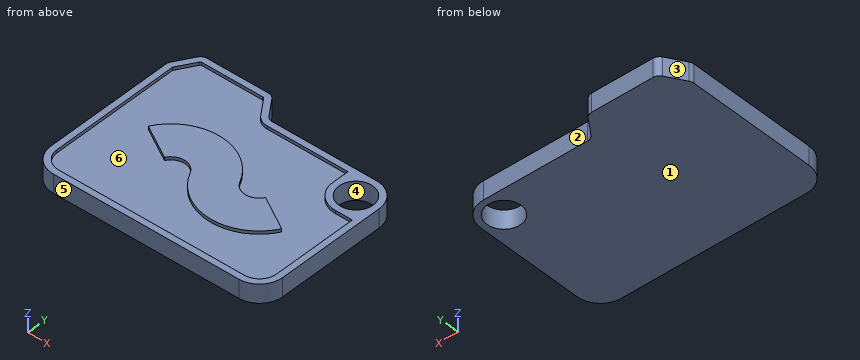
from build123d import *

# Parameters (mm, degrees)
F0_R     = 2.1999998258
F1_DEPTH = 2
F2_DEPTH = 0.4


# Not quite as in the source:
# - ends of sketch curves that miss each other by under 0.0002 mm in the source are joined


with BuildPart() as f1:
    # F0 (on Top) → F1 (new body)
    with BuildSketch(Plane.XY):
        with BuildLine():
            Line((12, 10), (-1.4882636307, 10))
            ThreePointArc((-1.4882636307, 10), (-1.9438159565, 10.1097909917), (-2.2993371991, 10.4150558431))
            Line((-2.2993371991, 10.4150558431), (-3.8642550313, 12.5849441569))
            ThreePointArc((-3.8642550313, 12.5849441569), (-4.2197762739, 12.8902090083), (-4.6753285997, 13))
            Line((-4.6753285997, 13), (-12.6032477109, 13))
            ThreePointArc((-12.6032477109, 13), (-13.0920798627, 12.8723778582), (-13.456140402, 12.5220862548))
            Line((-13.456140402, 12.5220862548), (-14.8528926911, 10.2403180459))
            ThreePointArc((-14.8528926911, 10.2403180459), (-14.9625208286, 9.989439561), (-15, 9.7182317911))
            Line((-15, 9.7182317911), (-15, -7))
            ThreePointArc((-15, -7), (-14.1213203436, -9.1213203436), (-12, -10))
            Line((-12, -10), (12, -10))
            ThreePointArc((12, -10), (14.1213203436, -9.1213203436), (15, -7))
            Line((15, -7), (15, 7))
            ThreePointArc((15, 7), (14.1213203436, 9.1213203436), (12, 10))
        make_face()
        with BuildLine():
            ThreePointArc((-14.1999998258, 9.7182317911), (-14.192503998, 9.7724732978), (-14.1705783896, 9.8226489511))
            Line((-14.1705783896, 9.8226489511), (-12.7738261005, 12.10441716))
            ThreePointArc((-12.7738261005, 12.10441716), (-12.7010140561, 12.1744754196), (-12.6032477109, 12.1999998258))
            Line((-12.6032477109, 12.1999998258), (-4.6753285997, 12.1999998258))
            ThreePointArc((-4.6753285997, 12.1999998258), (-4.5842182139, 12.1780416465), (-4.5131140273, 12.1169887295))
            Line((-4.5131140273, 12.1169887295), (-2.9481961951, 9.9471004156))
            ThreePointArc((-2.9481961951, 9.9471004156), (-2.3082578965, 9.3976236299), (-1.4882636307, 9.1999998258))
            Line((-1.4882636307, 9.1999998258), (9.0000001742, 9.1999998258))
            Line((9.0000001742, 9.1999998258), (9.0000001742, 7))
            ThreePointArc((9.0000001742, 7), (9.8786797797, 4.8786797797), (12, 4.0000001742))
            Line((12, 4.0000001742), (14.1999998258, 4))
            Line((14.1999998258, 4), (14.1999998258, -7))
            ThreePointArc((14.1999998258, -7), (13.5556347954, -8.5556347954), (12, -9.1999998258))
            Line((12, -9.1999998258), (-12, -9.1999998258))
            ThreePointArc((-12, -9.1999998258), (-13.5556347954, -8.5556347954), (-14.1999998258, -7))
            Line((-14.1999998258, -7), (-14.1999998258, 9.7182317911))
        make_face(mode=Mode.SUBTRACT)
        with Locations((12, 7)):
            Circle(F0_R, mode=Mode.SUBTRACT)
        with BuildLine():
            Line((-12.7738261005, 12.10441716), (-14.1705783896, 9.8226489511))
            ThreePointArc((-14.1705783896, 9.8226489511), (-14.192503998, 9.7724732978), (-14.1999998258, 9.7182317911))
            Line((-14.1999998258, 9.7182317911), (-14.1999998258, -7))
            ThreePointArc((-14.1999998258, -7), (-13.5556347954, -8.5556347954), (-12, -9.1999998258))
            Line((-12, -9.1999998258), (12, -9.1999998258))
            ThreePointArc((12, -9.1999998258), (13.5556347954, -8.5556347954), (14.1999998258, -7))
            Line((14.1999998258, -7), (14.1999998258, 4))
            Line((14.1999998258, 4), (12, 4))
            ThreePointArc((12, 4), (9.8786797797, 4.8786797797), (9.0000001742, 7))
            Line((9.0000001742, 7), (9.0000001742, 9.1999998258))
            Line((9.0000001742, 9.1999998258), (-1.4882636307, 9.1999998258))
            ThreePointArc((-1.4882636307, 9.1999998258), (-2.3082578965, 9.3976236299), (-2.9481961951, 9.9471004156))
            Line((-2.9481961951, 9.9471004156), (-4.5131140273, 12.1169887295))
            ThreePointArc((-4.5131140273, 12.1169887295), (-4.5842182139, 12.1780416465), (-4.6753285997, 12.1999998258))
            Line((-4.6753285997, 12.1999998258), (-12.6032477109, 12.1999998258))
            ThreePointArc((-12.6032477109, 12.1999998258), (-12.7010140561, 12.1744754196), (-12.7738261005, 12.10441716))
        make_face()
        with BuildLine():
            ThreePointArc((10, -1.5313274312), (3.7431454959, -4.9955321683), (-2.2491392669, -1.0915001412))
            ThreePointArc((-2.2491392669, -1.0915001412), (-3.9225638289, -0.0012477009), (-5.6698729811, -0.9686725688))
            Line((-5.6698729811, -0.9686725688), (-10, 1.5313274312))
            ThreePointArc((-10, 1.5313274312), (-3.7431454959, 4.9955321683), (2.2491392669, 1.0915001412))
            ThreePointArc((2.2491392669, 1.0915001412), (3.9225638289, 0.0012477009), (5.6698729811, 0.9686725688))
            Line((5.6698729811, 0.9686725688), (10, -1.5313274312))
        make_face(mode=Mode.SUBTRACT)
        with BuildLine():
            ThreePointArc((-5.6698729811, -0.9686725688), (-3.9225638289, -0.0012477009), (-2.2491392669, -1.0915001412))
            ThreePointArc((-2.2491392669, -1.0915001412), (3.7431454959, -4.9955321683), (10, -1.5313274312))
            Line((10, -1.5313274312), (5.6698729811, 0.9686725688))
            ThreePointArc((5.6698729811, 0.9686725688), (3.9225638289, 0.0012477009), (2.2491392669, 1.0915001412))
            ThreePointArc((2.2491392669, 1.0915001412), (-3.7431454959, 4.9955321683), (-10, 1.5313274312))
            Line((-10, 1.5313274312), (-5.6698729811, -0.9686725688))
        make_face()
    extrude(amount=-F1_DEPTH)

    # F0 (on Top) → F2 (join)
    with BuildSketch(Plane.XY):
        with BuildLine():
            Line((12, 10), (-1.4882636307, 10))
            ThreePointArc((-1.4882636307, 10), (-1.9438159565, 10.1097909917), (-2.2993371991, 10.4150558431))
            Line((-2.2993371991, 10.4150558431), (-3.8642550313, 12.5849441569))
            ThreePointArc((-3.8642550313, 12.5849441569), (-4.2197762739, 12.8902090083), (-4.6753285997, 13))
            Line((-4.6753285997, 13), (-12.6032477109, 13))
            ThreePointArc((-12.6032477109, 13), (-13.0920798627, 12.8723778582), (-13.456140402, 12.5220862548))
            Line((-13.456140402, 12.5220862548), (-14.8528926911, 10.2403180459))
            ThreePointArc((-14.8528926911, 10.2403180459), (-14.9625208286, 9.989439561), (-15, 9.7182317911))
            Line((-15, 9.7182317911), (-15, -7))
            ThreePointArc((-15, -7), (-14.1213203436, -9.1213203436), (-12, -10))
            Line((-12, -10), (12, -10))
            ThreePointArc((12, -10), (14.1213203436, -9.1213203436), (15, -7))
            Line((15, -7), (15, 7))
            ThreePointArc((15, 7), (14.1213203436, 9.1213203436), (12, 10))
        make_face()
        with BuildLine():
            ThreePointArc((-14.1999998258, 9.7182317911), (-14.192503998, 9.7724732978), (-14.1705783896, 9.8226489511))
            Line((-14.1705783896, 9.8226489511), (-12.7738261005, 12.10441716))
            ThreePointArc((-12.7738261005, 12.10441716), (-12.7010140561, 12.1744754196), (-12.6032477109, 12.1999998258))
            Line((-12.6032477109, 12.1999998258), (-4.6753285997, 12.1999998258))
            ThreePointArc((-4.6753285997, 12.1999998258), (-4.5842182139, 12.1780416465), (-4.5131140273, 12.1169887295))
            Line((-4.5131140273, 12.1169887295), (-2.9481961951, 9.9471004156))
            ThreePointArc((-2.9481961951, 9.9471004156), (-2.3082578965, 9.3976236299), (-1.4882636307, 9.1999998258))
            Line((-1.4882636307, 9.1999998258), (9.0000001742, 9.1999998258))
            Line((9.0000001742, 9.1999998258), (9.0000001742, 7))
            ThreePointArc((9.0000001742, 7), (9.8786797797, 4.8786797797), (12, 4.0000001742))
            Line((12, 4.0000001742), (14.1999998258, 4))
            Line((14.1999998258, 4), (14.1999998258, -7))
            ThreePointArc((14.1999998258, -7), (13.5556347954, -8.5556347954), (12, -9.1999998258))
            Line((12, -9.1999998258), (-12, -9.1999998258))
            ThreePointArc((-12, -9.1999998258), (-13.5556347954, -8.5556347954), (-14.1999998258, -7))
            Line((-14.1999998258, -7), (-14.1999998258, 9.7182317911))
        make_face(mode=Mode.SUBTRACT)
        with Locations((12, 7)):
            Circle(F0_R, mode=Mode.SUBTRACT)
        with BuildLine():
            ThreePointArc((-5.6698729811, -0.9686725688), (-3.9225638289, -0.0012477009), (-2.2491392669, -1.0915001412))
            ThreePointArc((-2.2491392669, -1.0915001412), (3.7431454959, -4.9955321683), (10, -1.5313274312))
            Line((10, -1.5313274312), (5.6698729811, 0.9686725688))
            ThreePointArc((5.6698729811, 0.9686725688), (3.9225638289, 0.0012477009), (2.2491392669, 1.0915001412))
            ThreePointArc((2.2491392669, 1.0915001412), (-3.7431454959, 4.9955321683), (-10, 1.5313274312))
            Line((-10, 1.5313274312), (-5.6698729811, -0.9686725688))
        make_face()
    extrude(amount=F2_DEPTH)


solid = f1.part
Can you work these out from the model? Positions are in its coordinate system, mm. Face numbers are marked on the shaded views. A direction names the side the tool comes from. Round coordinates to 2 decimals unless told otherwise and drop trailing zeros. Write each loop counter-clockwise with the first axis right and the second up, starting at its lowest first coordinate (ties: lowest second). Pieces come first, ordered by that corner, then holes. Notation, with made-up numbers: (75, 63.25) -> (127, 63.25) arc R29 ccw to (127, 88.25) -> close; hole circle Ø2 at (-3.75, -35). An arc over 180 degrees is marked (long way). Use one line per item in the form item = value. Start each with the question number.
Q1. Imagine slicing it at B-B (y = 8). Please give me the cut outline in (x, z), then the cut area to 3 significant figures.
Q2. Imagine slicing it at C-C (x = -7.5). Please give me the cut outline in (y, z).
Q3. I'm going to push flat-ended pins straight in: P1, Ø1, axis at x = 9.5, y = 2.5, coming from the +Z side; P2, Ø1.2, axis at x = 8, z = -0.5, coming from the +Y side; P3, Ø8, axis at x = -7, y = -0.5, coming from the +Z side. Where does each tip first touch, or does it pass through?
Q4. We'd pull the mould along Y, two halves only. Please class the marked faces 3, 4, 5 and 6: +Y half, -Y half, draft (parallel to the pull), parting line (faces both ways), or undercut.
Q5. If I drill on probe 1 along Y at (x, z) = (12, -0.4); probe 2 along Z at (x, y) = (-1, 4.75); probe 3 along Y at (x, z) = (-9, 0.05), over which ranges is the centre line in solid material (lowest first)? Write a range as [from, to].
Q6. Which directions (+Z, -Z, +X, -X, +Y, -Y) give clear straight access to the entire face, cutting with the end or side of a thin tool? Please do the marked faces 1 and 2.
Q7. Imagine slicing it at A-A (z = -0.75). Please give me the cut outline in (x, y).
Q8. Imagine slicing it at D-D (y = -8). Please give me the cut outline in (x, z).
Worked out:
q1.outline = (-15, -2) -> (10.04, -2) -> (10.04, 0.4) -> (9, 0.4) -> (9, 0) -> (-14.2, 0) -> (-14.2, 0.4) -> (-15, 0.4) -> close; (13.96, -2) -> (14.83, -2) -> (14.83, 0.4) -> (13.96, 0.4) -> close
q1.area = 52.9 mm^2
q2.outline = (-10, -2) -> (13, -2) -> (13, 0.4) -> (12.2, 0.4) -> (12.2, 0) -> (4.05, 0) -> (4.05, 0.4) -> (0.09, 0.4) -> (0.09, 0) -> (-9.2, 0) -> (-9.2, 0.4) -> (-10, 0.4) -> close
q3.P1 = 0
q3.P2 = 10
q3.P3 = 0.4
q4.face_3 = +Y half
q4.face_4 = undercut
q4.face_5 = -Y half
q4.face_6 = undercut
q5.probe_1 = [-10, 4.8], [9.2, 10]
q5.probe_2 = [-2, 0]
q5.probe_3 = [-10, -9.2], [0.95, 2.86], [12.2, 13]
q6.face_1 = -Z, +X, -X, +Y, -Y
q6.face_2 = +Z, -Z, +X, +Y
q7.outline = (-15, -7) arc R3 ccw to (-12, -10) -> (12, -10) arc R3 ccw to (15, -7) -> (15, 7) arc R3 ccw to (12, 10) -> (-1.49, 10) arc R1 cw to (-2.3, 10.42) -> (-3.86, 12.58) arc R1 ccw to (-4.68, 13) -> (-12.6, 13) arc R1 ccw to (-13.46, 12.52) -> (-14.85, 10.24) arc R1 ccw to (-15, 9.72) -> close; hole circle Ø4.4 at (12, 7)
q8.outline = (-14.83, -2) -> (14.83, -2) -> (14.83, 0.4) -> (13.96, 0.4) -> (13.96, 0) -> (-13.96, 0) -> (-13.96, 0.4) -> (-14.83, 0.4) -> close
